from build123d import *

# Parameters (mm, degrees)
SKETCH1_W           = 80
SKETCH1_H           = 62
BOSS_EXTRUDE1_DEPTH = 3.7
SKETCH2_W           = 10
SKETCH2_H           = 20
BOSS_EXTRUDE2_DEPTH = 10
FILLET1_R           = 2
FILLET2_R           = 2


with BuildPart() as part:
    # Sketch1 → Boss-Extrude1 (new body)
    with BuildSketch(Plane(origin=(0, 0, 0), x_dir=(1, 0, 0), z_dir=(0, 1, 0))):
        with Locations((40, 31)):
            Rectangle(SKETCH1_W, SKETCH1_H)
    extrude(amount=BOSS_EXTRUDE1_DEPTH)

    # Sketch2 → Boss-Extrude2 (add)
    with BuildSketch(Plane(origin=(0, 3.7, 0), x_dir=(1, 0, 0), z_dir=(0, 1, 0))):
        with Locations((40, 31)):
            Rectangle(SKETCH2_W, SKETCH2_H)
    extrude(amount=BOSS_EXTRUDE2_DEPTH)

    # Fillet1
    fillet1_edges = [part.edges().sort_by_distance(p)[0] for p in [
        (35, 3.7, -31),
        (40, 3.7, -21),
        (45, 3.7, -31),
        (40, 3.7, -41),
    ]]
    fillet(fillet1_edges, radius=FILLET1_R)

    # Fillet2
    fillet2_edges = [part.edges().sort_by_distance(p)[0] for p in [
        (35, 13.7, -31),
        (40, 13.7, -21),
        (45, 13.7, -31),
        (40, 13.7, -41),
    ]]
    fillet(fillet2_edges, radius=FILLET2_R)


solid = part.part
CAD build for the part. Positions are in the model's coordinates, mm. A direction names the side the tool comes from. Coordinates: 2 decimals unless noted, no trailing zeros. Order: outer loops, then holes, each group sorted by start corner. A loop starts at its lowest first (then second) coordinate and runs counter-clockwise, first axis right, second up. Notation, with made-up numbers: (-39, -27) -> (8, -27) arc R16 ccw to (8, -15) -> close; hole circle Ø4 at (72.25, 81). An arc over 180 degrees is marked (long way). Answer in a Markdown table with one row per item.
1) Drill centre lines: line 1 (Y direction, x = 28.5, z = -52); line 2 (X direction, y = 11.25, z = -30); line 3 (Z direction, x = 44, y = 8.75). Where is each one in solid material? Low to high.
Check values:
| item | result |
|---|---|
| line 1 | 0 to 3.7 |
| line 2 | 35 to 45 |
| line 3 | -41 to -21 |
2) Band-saw the part on A-A (z = -37). List the corners of the cut face in (x, y).
Check values:
| item | result |
|---|---|
| outline | (0, 0) -> (80, 0) -> (80, 3.7) -> (47, 3.7) arc R2 cw to (45, 5.7) -> (45, 11.7) arc R2 ccw to (43, 13.7) -> (37, 13.7) arc R2 ccw to (35, 11.7) -> (35, 5.7) arc R2 cw to (33, 3.7) -> (0, 3.7) -> close |
3) Flat gauge pins, fed straight in: P1, Ø8, axis at x = 59.5, z = -30.5, coming from the +Y side; P2, Ø3, axis at y = 7.5, z = -30.5, coming from the -X side; P3, Ø1.8, axis at x = 41.5, y = 8, coming from the +Z side. Where does each tip first touch, or does it go through?
Check values:
| item | result |
|---|---|
| P1 | y = 3.7 |
| P2 | x = 35 |
| P3 | z = -21 |
4) Band-saw the part on C-C (y = 10.5). List the corners of the cut face in (x, z).
Check values:
| item | result |
|---|---|
| outline | (35, -41) -> (45, -41) -> (45, -21) -> (35, -21) -> close |
5) Band-saw the part on D-D (z = -14.5). List the corners of the cut face in (x, y), and give its area (3 significant figures).
Check values:
| item | result |
|---|---|
| outline | (0, 0) -> (80, 0) -> (80, 3.7) -> (0, 3.7) -> close |
| area | 296 mm2 |
6) Which spindle directions (+Z, -Z, +X, -X, +Y, -Y) get a long thin tool onto all of the face, cutting with end or side? Do faces 1 (the face through (45, 9, -31)), 2 (the face through (35, 9, -31)), 3 (the face through (40, 9, -21)), 4 (the face through (40, 9, -41)). Say none if no direction does.
Check values:
| item | result |
|---|---|
| face 1 | +Z, -Z, +X, +Y |
| face 2 | +Z, -Z, -X, +Y |
| face 3 | +Z, +X, -X, +Y |
| face 4 | -Z, +X, -X, +Y |
7) Band-saw the part on B-B (x = 40.5). List the corners of the cut face in (y, z), and give its area (3 significant figures).
Check values:
| item | result |
|---|---|
| outline | (0, -62) -> (3.7, -62) -> (3.7, -43) arc R2 cw to (5.7, -41) -> (11.7, -41) arc R2 ccw to (13.7, -39) -> (13.7, -23) arc R2 ccw to (11.7, -21) -> (5.7, -21) arc R2 cw to (3.7, -19) -> (3.7, 0) -> (0, 0) -> close |
| area | 429 mm2 |
